Build history of the part. All positions in model axes, mm. Round coordinates to 2 decimals unless told otherwise and drop trailing zeros. Order: outer loops, then holes, each group sorted by start corner. A loop starts at its lowest first (then second) coordinate and runs counter-clockwise, first axis right, second up. Notation, with made-up numbers: (0.5, 25.25) -> (12.5, 25.25) arc R13 ccw to (12.5, 38.25) -> close; hole circle Ø10 at (48, -18). An arc over 180 degrees is marked (long way). Answer as CSV lines item,"result". Start each with the question number.
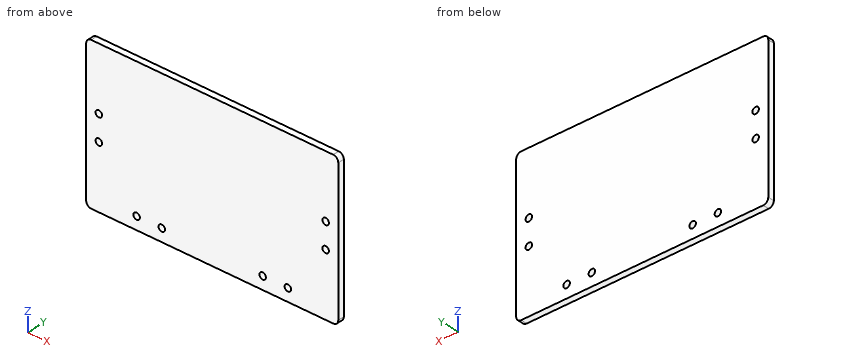
```python
from build123d import *

# Parameters (mm, degrees)
SKETCH1_W           = 254
SKETCH1_H           = 152.4
BOSS_EXTRUDE1_DEPTH = 6.35
SKETCH3_R           = 3.2639
CUT_EXTRUDE2_DEPTH  = 149.24224263
FILLET1_R           = 5.08


with BuildPart() as part:
    # Sketch1 → Boss-Extrude1 (new body)
    with BuildSketch(Plane(origin=(0, 0, 0), x_dir=(1, 0, 0), z_dir=(0, 1, 0))):
        Rectangle(SKETCH1_W, SKETCH1_H)
    extrude(amount=BOSS_EXTRUDE1_DEPTH)

    # Sketch3 → Cut-Extrude2 (cut, through all)
    with BuildSketch(Plane(origin=(0, 6.35, 0), x_dir=(1, 0, 0), z_dir=(0, 1, 0))):
        with Locations(Location((-114.3, 12.7, 0), (0, 0, 270))):
            Circle(SKETCH3_R)
        with Locations(Location((-114.3, -12.7, 0), (0, 0, 270))):
            Circle(SKETCH3_R)
        with Locations(Location((-76.2, 63.5, 0), (0, 0, 270))):
            Circle(SKETCH3_R)
        with Locations(Location((-50.8, 63.5, 0), (0, 0, 270))):
            Circle(SKETCH3_R)
        with Locations(Location((50.8, 63.5, 0), (0, 0, 90))):
            Circle(SKETCH3_R)
        with Locations(Location((76.2, 63.5, 0), (0, 0, 90))):
            Circle(SKETCH3_R)
        with Locations(Location((114.3, -12.7, 0), (0, 0, 90))):
            Circle(SKETCH3_R)
        with Locations(Location((114.3, 12.7, 0), (0, 0, 90))):
            Circle(SKETCH3_R)
    extrude(amount=-CUT_EXTRUDE2_DEPTH, mode=Mode.SUBTRACT)

    # Fillet1
    fillet1_edges = [part.edges().sort_by_distance(p)[0] for p in [
        (127, 3.175, 76.2),
        (-127, 3.175, 76.2),
        (-127, 3.175, -76.2),
        (127, 3.175, -76.2),
    ]]
    fillet(fillet1_edges, radius=FILLET1_R)


solid = part.part
```
Q1. Slice it at A-A, the plane z = 12.7. Write the cut outline in (x, y), plus the area to 3 significant figures.
Q2. Probe L1, parallel to X at y = 3, z = -63.5; L2, parallel to X at y = 1, z = 12.5; L3, parallel to Z at x = 50.8, y = 3.25. List the from-to ranges inside material, lowest first.
Q3. Slice it at B-B, the plane x = -76.2. Write the cut outline in (y, z).
Q4. Slice it at D-D, the plane x = -114.3. Write the cut outline in (y, z), plus the area to 3 significant figures.
Q5. Slice it at C-C, the plane z = -63.5. Write the cut outline in (x, y), plus the area to 3 significant figures.
Solutions:
1,outline,"(-127, 0) -> (-117.56, 0) -> (-117.56, 6.35) -> (-127, 6.35) -> close; (-111.04, 0) -> (111.04, 0) -> (111.04, 6.35) -> (-111.04, 6.35) -> close; (117.56, 0) -> (127, 0) -> (127, 6.35) -> (117.56, 6.35) -> close"
1,area,"1,530 mm2"
2,L1,"x = -127 to -79.46, -72.94 to -54.06, -47.54 to 47.54, 54.06 to 72.94, 79.46 to 127"
2,L2,"x = -127 to -117.56, -111.04 to 111.04, 117.56 to 127"
2,L3,"z = -76.2 to -66.76, -60.24 to 76.2"
3,outline,"(0, -76.2) -> (6.35, -76.2) -> (6.35, -66.76) -> (0, -66.76) -> close; (0, -60.24) -> (6.35, -60.24) -> (6.35, 76.2) -> (0, 76.2) -> close"
4,outline,"(0, -76.2) -> (6.35, -76.2) -> (6.35, -15.96) -> (0, -15.96) -> close; (0, -9.44) -> (6.35, -9.44) -> (6.35, 9.44) -> (0, 9.44) -> close; (0, 15.96) -> (6.35, 15.96) -> (6.35, 76.2) -> (0, 76.2) -> close"
4,area,"885 mm2"
5,outline,"(-127, 0) -> (-79.46, 0) -> (-79.46, 6.35) -> (-127, 6.35) -> close; (-72.94, 0) -> (-54.06, 0) -> (-54.06, 6.35) -> (-72.94, 6.35) -> close; (-47.54, 0) -> (47.54, 0) -> (47.54, 6.35) -> (-47.54, 6.35) -> close; (54.06, 0) -> (72.94, 0) -> (72.94, 6.35) -> (54.06, 6.35) -> close; (79.46, 0) -> (127, 0) -> (127, 6.35) -> (79.46, 6.35) -> close"
5,area,"1,450 mm2"
